Study the drawing (mm; zero at the part's minimum x, y, z) and answer. A direction names the side the tool comes from. Give positions to 0.01 mm unless a question says otherwise; leave off trailing zeros. Write each loop counter-clockwise with the first axis right and the second up, starting at its lowest first coordinate (ties: lowest second). Pieces come first, ordered by that corner, then holes. Notation, with made-up numbers: (60, 58) - (107, 58) arc R15 ccw to (107, 83) - close; hole circle Ø11 at (35.5, 63). An arc over 180 degrees is marked (long way). Return JSON: item names as keys, results as strings.
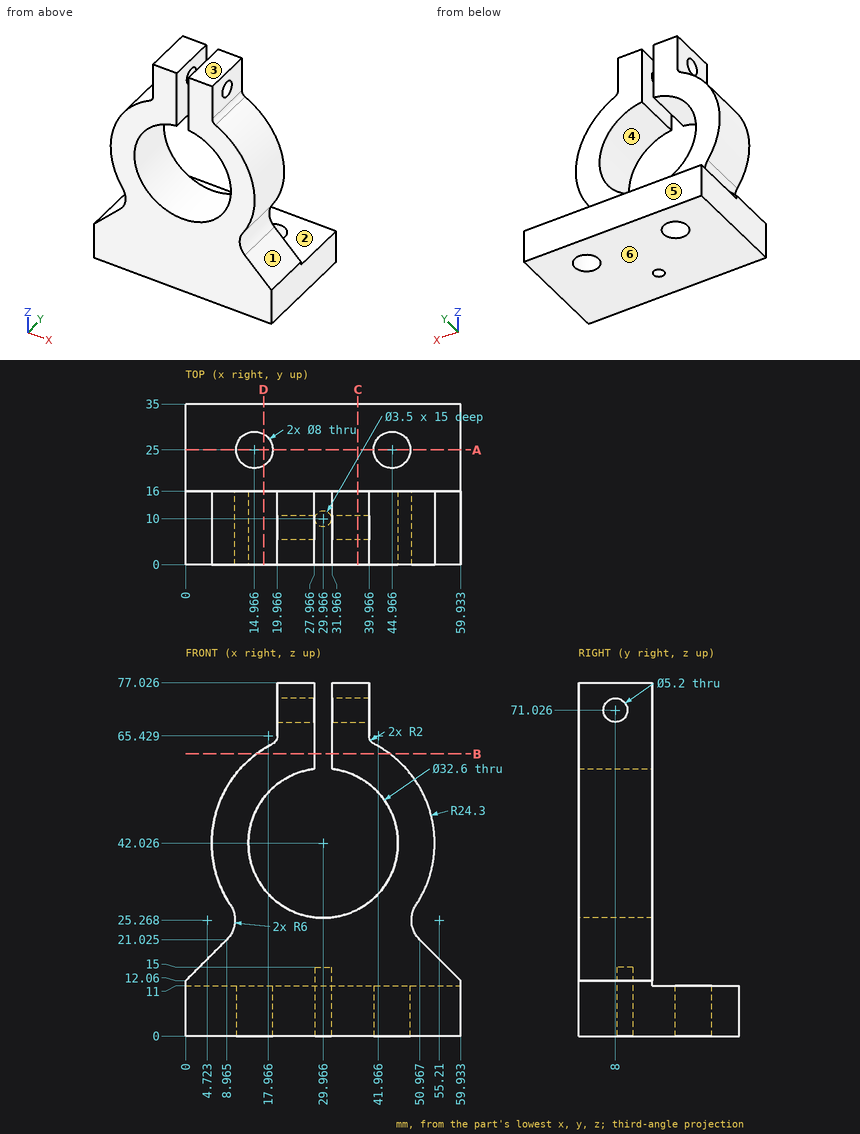
Item 1: A cutting plane is placed at D-D on x = 17. Determine the outline of the cut face in (y, z) (1 decimal).
Answer below:
{"outline": "(0, 0) - (21.6, 0) - (21.6, 11) - (16, 11) - (16, 32.1) - (0, 32.1) - close; (0, 51.9) - (16, 51.9) - (16, 62.6) - (0, 62.6) - close; (28.4, 0) - (35, 0) - (35, 11) - (28.4, 11) - close"}
Item 2: Consider L1, parallel to Z at x = 21.5, y = 8 (1 decimal); L2, parallel to Y at x = 15, z = 3.5; L3, parallel to Z at x = 34, y = 9 (1 decimal). Determine where each line is inside the solid, lowest interval first.
Answer below:
{"L1": "z = 0 to 28.1, 56 to 68.4, 73.6 to 77", "L2": "y = 0 to 21, 29 to 35", "L3": "z = 0 to 26.2, 57.8 to 68.6, 73.4 to 77"}
Item 3: A cutting plane is placed at A-A on y = 25. Determine the outline of the cut face in (x, z).
Answer below:
{"outline": "(0, 0) - (10.97, 0) - (10.97, 11) - (0, 11) - close; (18.97, 0) - (40.97, 0) - (40.97, 11) - (18.97, 11) - close; (48.97, 0) - (59.93, 0) - (59.93, 11) - (48.97, 11) - close"}
Item 4: A cutting plane is placed at B-B on z = 61.5. Determine the outline of the cut face in (x, y).
Answer below:
{"outline": "(15.43, 0) - (27.97, 0) - (27.97, 16) - (15.43, 16) - close; (31.97, 0) - (44.5, 0) - (44.5, 16) - (31.97, 16) - close"}
Item 5: The mould has two halves that part along Z. Classify the marked faces 4, 5 and 6: +Z half, -Z half, draft (parallel to the pull), parting line (faces both ways), or undercut.
Answer below:
{"face 4": "undercut", "face 5": "draft", "face 6": "-Z half"}
Item 6: Flat-ended cylindrical pins translate along their axes: P1, Ø17.5, axis at y = 6.5, z = 69.5, coming from the +X side (1 decimal); P2, Ø5.5, axis at x = 28, y = 21, coming from the +Z side; P3, Ø5, axis at y = 8, z = 68.5, coming from the -X side; P4, Ø4, axis at x = 30.5, y = 10.5, coming from the -Z side. Find the tip coordinate at first contact, or state that the pin passes through.
Answer below:
{"P1": "stops at x = 45.5", "P2": "stops at z = 11", "P3": "stops at x = 19.97", "P4": "stops at z = 0"}
Item 7: A cutting plane is placed at C-C on x = 37.5. Determine the outline of the cut face in (y, z).
Answer below:
{"outline": "(0, 0) - (35, 0) - (35, 11) - (16, 11) - (16, 27.57) - (0, 27.57) - close; (0, 56.48) - (16, 56.48) - (16, 77.03) - (0, 77.03) - close; hole circle Ø5.2 at (8, 71.03)"}
Item 8: For the marked faces 1, 2 and 3, determine the directions among +Z, -Z, +X, -X, +Y, -Y from which every point of the face is accessible in a straight line to the end or side of a thin tool.
Answer below:
{"face 1": "+X, +Y, -Y", "face 2": "+Z, +X, -X, +Y", "face 3": "+Z, +X, -X, +Y, -Y"}
